Read the model definition and answer for the solid it produces. Units are mm, in the model's axes. A direction names the side the tool comes from. Give positions to 0.01 mm unless a question says otherwise; leave off trailing zeros. Order: outer loops, then holes, each group sorted by start corner. A loop starts at its lowest first (then second) coordinate and runs counter-clockwise, first axis right, second up. Notation, with made-up numbers: M -1.5,1.5 L 41.5,1.5 A28 cw 41.5,34.5 Z; hole C 84.5,69.5 d9. An arc over 180 degrees is marked long. One line per item, written item: value.
from build123d import *

# Parameters (mm, degrees)
EXTRUDE_1_DEPTH     = 15
CHAMFER_1_SIZE      = 2
CHAMFER_2_SIZE      = 0.5
MIRROR_START        = -9.237604307
MIRROR_2_DEPTH      = 2.598076211
MIRROR_START_2      = 6.639528096
MIRROR_2_2_DEPTH    = 2.598076211
SKETCH_2_R          = 1.5
CUT_EXTRUDE_1_DEPTH = 1


# Read off the part's stored shape, not the designer's step: 镜向2
with BuildPart() as part:
    # 草图1 → 凸台-拉伸1 (new, symmetric)
    with BuildSketch(Plane.XY):
        Polygon((-3, 0), (3, 0), (3, -3), (5.3, -3), (5.3, -7), (-5.3, -7), (-5.3, -3), (-3, -3), align=None)
    extrude(amount=EXTRUDE_1_DEPTH, both=True)

    # 倒角1
    chamfer_1_edges = [part.edges().sort_by_distance(p)[0] for p in [
        (5.3, -7, 0),
        (-5.3, -7, 0),
    ]]
    chamfer(chamfer_1_edges, length=CHAMFER_1_SIZE)

    # 倒角2
    chamfer_2_edges = [part.edges().sort_by_distance(p)[0] for p in [
        (-3, -1.5, 15),
        (-4.15, -3, 15),
        (-5.3, -4, 15),
        (5.3, -4, 15),
        (4.15, -3, 15),
        (3, -1.5, 15),
    ]]
    chamfer(chamfer_2_edges, length=CHAMFER_2_SIZE)

    # 镜向2 outline → 镜向2 (cut)
    with BuildSketch(Plane(origin=(0, 0, 0), x_dir=(0.816496580927727, -0.4082482904638606, -0.4082482904638635), z_dir=(0.5773502691896244, 0.5773502691896244, 0.5773502691896285)).offset(MIRROR_START)):
        Polygon((9.593834826, 8.131727984), (11.471776962, 8.131727984), (12.288273543, 6.717514421), (13.279880956, 5), (14, 5), (14, 12), (7.360486936, 12), (8.164965809, 10.606601718), align=None)
    extrude(amount=MIRROR_2_DEPTH, mode=Mode.SUBTRACT)

    # Mirror 2 2 outline → Mirror 2 2 (cut)
    with BuildSketch(Plane(origin=(0, 0, 0), x_dir=(0.816496580927727, 0.4082482904638606, 0.4082482904638635), z_dir=(0.5773502691896244, -0.5773502691896244, -0.5773502691896285)).offset(MIRROR_START_2)):
        Polygon((-8.164965809, -10.606601718), (-9.593834826, -8.131727984), (-11.471776962, -8.131727984), (-12.288273543, -6.717514421), (-13.279880956, -5), (-14, -5), (-14, -12), (-7.360486936, -12), align=None)
    extrude(amount=MIRROR_2_2_DEPTH, mode=Mode.SUBTRACT)

    # 草图2 → 切除-拉伸1 (cut)
    with BuildSketch(Plane(origin=(0, 0, 0), x_dir=(1, 0, 0), z_dir=(0, 1, 0))):
        with Locations(Location((0, 9, 0), (0, 0, 270))):
            Circle(SKETCH_2_R)
        with Locations(Location((0, -9, 0), (0, 0, 90))):
            Circle(SKETCH_2_R)
    extrude(amount=-CUT_EXTRUDE_1_DEPTH, mode=Mode.SUBTRACT)


solid = part.part
1) Find section D-D, the plane x = -3.75. Write down the section's boundary in (y, z).
Reported:
outline: M -6.55,-15 L -3.5,-15 L -3,-14.5 L -3,14.5 L -3.5,15 L -6.55,15 Z
2) Which of the six approach directions +Z, -Z, +X, -X, +Y, -Y give full straight-line access (tool end or side, diameter ignored) to faces 4 (the face through (3, -1, 0)), 5 (the face through (-3, -2, 0)), 6 (the face through (0, -1, -9))?
Reported:
face 4: +Z, -Z, +X, +Y
face 5: +Z, -Z, -X, +Y
face 6: +Y
3) Determine the mould class of faces 1 (the face through (-4, -3, 0)), 2 (the face through (0, -4, -15)), 3 (the face through (-0.07, -0.49, 10.5)) for opening direction Z: +Z half, -Z half, draft (parallel to the pull), parting line (faces both ways), or undercut.
Reported:
face 1: draft
face 2: -Z half
face 3: undercut
4) Find section A-A, the plane x = 0. Write down the section's boundary in (y, z).
Reported:
outline: M -7,-15 L 0,-15 L 0,-10.5 L -1,-10.5 L -1,-7.5 L 0,-7.5 L 0,7.5 L -1,7.5 L -1,10.5 L 0,10.5 L 0,15 L -7,15 Z
5) Find section B-B, the plane z = 11.5. Write down the section's boundary in (x, y), plus the area to 3 significant figures.
Reported:
outline: M -5.3,-5 L -3.3,-7 L 3.3,-7 L 5.3,-5 L 5.3,-3 L 3,-3 L 3,0 L -3,0 L -3,-3 L -5.3,-3 Z
area: 56.4 mm^2
6) Each of these flat-tipped pins is pushed along its axis until it touches: pin 1 Ø0.7 at (x, z) = (3.5, -4.5) entering from +Y; pin 2 Ø0.9 at (y, z) = (-2, -3.5) entering from -X; pin 3 Ø0.9 at (y, z) = (-1, -7) entering from +X. Where does it stop, or does it pass through?
Reported:
pin 1: stops at y = -3
pin 2: stops at x = -3
pin 3: stops at x = 3
7) Find section C-C, the plane y = -0.5. Write down the section's boundary in (x, z).
Reported:
outline: M -3,-14.5 L -2.5,-15 L 2.5,-15 L 3,-14.5 L 3,14.5 L 2.5,15 L -2.5,15 L -3,14.5 Z; hole C 0,-9 d3; hole C 0,9 d3
8) Consider probe 1 along X at (y, z) = (-0.35, 9); probe 2 along Y at (x, z) = (-0.5, -8.5); probe 3 along X at (y, z) = (-2.5, 3). Determine where each line is inside the solid, lowest interval first.
Reported:
probe 1: x = -3 to -1.5, 1.5 to 3
probe 2: y = -7 to -1
probe 3: x = -3 to 3
